For this review, take the finished solid that the model builds, in its own axes (mm). A direction names the side the tool comes from. Give positions to 0.01 mm unless a question says otherwise; leave off trailing zeros. Loops run counter-clockwise (first coordinate to the right, second up) from the corner with the lowest first, then second, coordinate; pieces in that order, holes last.
Autodesk Inventor part; units mm, degrees
ref_plane "YZ Plane" through (0, 0, 0) normal (1, 0, 0) x (0, 1, 0)
ref_plane "XZ Plane" through (0, 0, 0) normal (0, 1, 0) x (-1, 0, 0)
ref_plane "XY Plane" through (0, 0, 0) normal (0, 0, 1) x (1, 0, 0)
sketch "Sketch1" plane through (0, 0, 0) normal (1, 0, 0) x (0, 1, 0)
  line L0 (-91.985, -4.7571) -> (-89.0815, -4.7571)
  line L1 (-89.0815, -4.7571) -> (-89.0815, -7.1749)
  line L2 (-89.0815, -7.1749) -> (-81.5711, -7.1749)
  line L3 (-57.4992, -7.1749) -> (-57.4992, -4.7571)
  line L4 (-57.4992, -4.7571) -> (-54.5957, -4.7571)
  line L5 (-54.5957, -4.7571) -> (-54.5957, -4.795)
  line L6 (-54.5957, -4.795) -> (-53.1756, -4.795)
  line L7 (-53.1756, -4.795) -> (-53.1756, 8.1844)
  line L8 (-53.1756, 8.1844) -> (-54.5957, 8.1844)
  line L9 (-54.5957, 8.1844) -> (-54.5957, 8.1465)
  line L10 (-54.5957, 8.1465) -> (-57.4992, 8.1465)
  line L11 (-57.4992, 8.1465) -> (-57.4992, 10.5643)
  line L12 (-57.4992, 10.5643) -> (-61.7845, 10.5643)
  line L13 (-89.0815, 10.5643) -> (-89.0815, 8.1465)
  line L14 (-89.0815, 8.1465) -> (-91.985, 8.1465)
  line L15 (-91.985, 8.1465) -> (-91.985, 8.1844)
  line L16 (-91.985, 8.1844) -> (-93.4052, 8.1844)
  line L17 (-93.4052, 8.1844) -> (-93.4052, -4.795)
  line L18 (-93.4052, -4.795) -> (-91.985, -4.795)
  line L19 (-91.985, -4.795) -> (-91.985, -4.7571)
  line L20 (-81.5711, 10.5643) -> (-89.0815, 10.5643)
  line L21 (-61.7845, -7.1749) -> (-57.4992, -7.1749)
  line L22 (-61.7845, 10.5643) -> (-81.5711, 10.5643)
  line L23 (-61.7845, -7.1749) -> (-81.5711, -7.1749)
  point P0 (0, 0)
extrude "Extrusion1" add sketch "Sketch1" along normal blind 2.921
Item 1: For L1, parallel to Y at x = 2.45, z = -5; L2, parallel to Z at x = 2.4, y = -89.5, list the stretches that pass through material, from the lowest coordinate up.
Answer:
L1: y = -89.08 to -57.5
L2: z = -4.76 to 8.15
Item 2: Take a section at B-B on y = -90. Give the boundary of the cut face in (x, z).
Answer:
outline: (0, -4.76) - (2.92, -4.76) - (2.92, 8.15) - (0, 8.15) - close
Item 3: Tool access review of faces 1 (the flat face through (1, -91, 8.146)), 2 (the flat face through (1, -93, 8.184)), 3 (the flat face through (1, -56, -4.757)), 4 (the flat face through (1, -93, -4.795)): name each direction out of +Z, -Z, +X, -X, +Y, -Y from which nothing blocks a thin tool from reaching the whole face with its end or side.
Answer:
face 1: +Z, +X, -X
face 2: +Z, +X, -X, -Y
face 3: -Z, +X, -X
face 4: -Z, +X, -X, -Y
Item 4: The part is to be moulded in two halves that separate along Y. For faces 5 (the flat face through (1, -53.176, 2)), 6 (the flat face through (2.921, -74, 2)), 7 (the flat face through (1, -91, -4.757)), 8 (the flat face through (1, -93.405, 2)), say which applies: released by +Y, released by -Y, zero draft, split by the parting line, or undercut.
Answer:
face 5: released by +Y
face 6: zero draft
face 7: undercut
face 8: released by -Y
Item 5: Clearance check with flat-ended pins moving along their axes: pin 1 Ø1.5 at (x, y) = (1.5, -91) entering from +Z; pin 2 Ø1.2 at (x, z) = (2, 9) entering from +Y; pin 3 Ø1.6 at (x, y) = (2, -92.5) entering from -Z (3 decimals). State where each tip first meets the part, or that it passes through.
Answer:
pin 1: stops at z = 8.15
pin 2: stops at y = -57.5
pin 3: stops at z = -4.795
